The model under review builds one solid part; all positions refer to its coordinate system, in mm. A direction names the side the tool comes from. Round coordinates to 2 decimals unless told otherwise and drop trailing zeros. Order: outer loops, then holes, each group sorted by start corner. A loop starts at its lowest first (then second) coordinate and runs counter-clockwise, first axis right, second up.
1) Consider section B-B (x = -6). Give the boundary of the cut face in (y, z).
2) Clearance check with flat-ended pins moving along their axes: P1, Ø1, axis at y = 6.5, z = 4, coming from the +X side; P2, Ø3.5, axis at x = 0, y = 6, coming from the -Z side; P3, Ø1, axis at x = 6, z = 2.5, coming from the -Y side; P4, Ø1.7, axis at x = 4.24, y = 4.24, coming from the +Z side. State where each tip first meets the part, or that it passes through.
3) To check wall thickness, follow L1, parallel to Y at x = 0, z = 3.25; L2, parallel to Y at x = 0, z = 4.9. State the ranges of each line that lie inside material, in increasing order.
4) Consider section C-C (x = -0.5). Give the boundary of the cut face in (y, z), then the cut area to 3 significant figures.
5) Mouldability with a two-part tool opening along Y and no side actions: class faces 4 (the face through (4, 2, 5.3)), 5 (the face through (3.757, 5.174, 3.019)), 6 (the face through (-2.87, -2.64, 0.39)) as pulls with the +Y half, pulls with the -Y half, needs draft (parallel to the pull), parting line crosses it, or undercut.
6) Machinability: for faces 1 (the face through (-2, 0, 4.2)), 2 (the face through (4, 2, 0.8)), 3 (the face through (7.04, -0.14, 3.02)), which of the approach directions +Z, -Z, +X, -X, +Y, -Y give a long, thin tool a straight path to every point of the face, cutting with its end or side? Answer none if there is none.
7) Consider section A-A (y = 0). Give the boundary of the cut face in (x, z).
from build123d import *

# Parameters (mm, degrees)
SKETCH_3_R               = 1.05
CUT_EXTRUDE_1_DEPTH      = 13.703149216
PATTERN_CIRCULAR_1_COUNT = 8


with BuildPart() as part:
    # ｽｹｯﾁ2 → 回転1 (revolve)
    with BuildSketch(Plane(origin=(0, 0, 0), x_dir=(1, 0, 0), z_dir=(0, 1, 0))):
        Polygon((3.9, 0), (1.5, 0), (1.5, -4.2), (4.15, -4.2), (4.15, -5.3), (8.4, -5.3), (8.4, -0.8), (3.9, -0.8), align=None)
    revolve(axis=Axis((0, 0, 4.2), (0, 0, -1)))

    # ｽｹｯﾁ3 → ｶｯﾄ - 押し出し1 (cut, through all)
    with BuildSketch(Plane(origin=(0, 0, 0.8), x_dir=(-1, 0, 0), z_dir=(0, 0, -1))):
        with Locations((0, 6)):
            Circle(SKETCH_3_R)
    cut_extrude_1 = extrude(amount=-CUT_EXTRUDE_1_DEPTH, mode=Mode.SUBTRACT)

    # 円形ﾊﾟﾀｰﾝ1: ｶｯﾄ - 押し出し1 ×8 about axis
    pattern_circular_1_axis = Axis((0, 0, 0), (0, 0, 1))
    for i in range(1, PATTERN_CIRCULAR_1_COUNT):
        add(cut_extrude_1.rotate(pattern_circular_1_axis, i * 360 / PATTERN_CIRCULAR_1_COUNT), mode=Mode.SUBTRACT)


solid = part.part
Answer below:
1. outline: (-5.88, 0.8) - (-1.05, 0.8) - (-1.05, 5.3) - (-5.88, 5.3) - close; (1.05, 0.8) - (5.88, 0.8) - (5.88, 5.3) - (1.05, 5.3) - close
2. P1: stops at x = 5.88
2. P2: stops at z = 0.8
2. P3: stops at y = -6.35
2. P4: passes through
3. L1: y = -8.4 to -7.05, -4.95 to -1.5, 1.5 to 4.95, 7.05 to 8.4
3. L2: y = -8.4 to -7.05, -4.95 to -4.15, 4.15 to 4.95, 7.05 to 8.4
4. outline: (-8.39, 0.8) - (-6.92, 0.8) - (-6.92, 5.3) - (-8.39, 5.3) - close; (-5.08, 0.8) - (-3.87, 0.8) - (-3.87, 0) - (-1.41, 0) - (-1.41, 4.2) - (-4.12, 4.2) - (-4.12, 5.3) - (-5.08, 5.3) - close; (1.41, 0) - (3.87, 0) - (3.87, 0.8) - (5.08, 0.8) - (5.08, 5.3) - (4.12, 5.3) - (4.12, 4.2) - (1.41, 4.2) - close; (6.92, 0.8) - (8.39, 0.8) - (8.39, 5.3) - (6.92, 5.3) - close
4. area: 44.1 mm2
5. face 4: needs draft
5. face 5: undercut
5. face 6: parting line crosses it
6. face 1: +Z
6. face 2: -Z
6. face 3: +Z, -Z
7. outline: (-8.4, 0.8) - (-7.05, 0.8) - (-7.05, 5.3) - (-8.4, 5.3) - close; (-4.95, 0.8) - (-3.9, 0.8) - (-3.9, 0) - (-1.5, 0) - (-1.5, 4.2) - (-4.15, 4.2) - (-4.15, 5.3) - (-4.95, 5.3) - close; (1.5, 0) - (3.9, 0) - (3.9, 0.8) - (4.95, 0.8) - (4.95, 5.3) - (4.15, 5.3) - (4.15, 4.2) - (1.5, 4.2) - close; (7.05, 0.8) - (8.4, 0.8) - (8.4, 5.3) - (7.05, 5.3) - close
